Design review of the part built by this model. Coordinates are the model's own, in mm. Face numbers are marked on the shaded views. A direction names the side the tool comes from. Round coordinates to 2 decimals unless told otherwise and drop trailing zeros. Order: outer loops, then holes, each group sorted by start corner. A loop starts at its lowest first (then second) coordinate and runs counter-clockwise, first axis right, second up. Notation, with made-up numbers: (59, -3.75) - (102, -3.75) arc R37 cw to (102, 33.25) - close; hole circle Ø4 at (59, 0.25). An arc over 180 degrees is marked (long way). Write item = value, one per line.
from build123d import *

# Parameters (mm, degrees)
F0_R     = 9.525
F1_DEPTH = 50.8
F2_SIZE  = 0.762
F3_W     = 9.525
F3_H     = 5.747142
F4_DEPTH = 12.7


with BuildPart() as f1:
    # F0 (on Front) → F1 (new body)
    with BuildSketch(Plane.XZ):
        Circle(F0_R)
    extrude(amount=-F1_DEPTH)

    # F2
    f2_edges = [f1.edges().sort_by_distance(p)[0] for p in [
        (-9.525, 0, 0),
        (-9.525, 50.8, 0),
    ]]
    chamfer(f2_edges, length=F2_SIZE)

    # F3 (on Right) → F4 (cut, symmetric)
    with BuildSketch(Plane.YZ):
        with Locations((12.7, 9.223571)):
            Rectangle(F3_W, F3_H)
        with Locations((38.1, 9.223571)):
            Rectangle(F3_W, F3_H)
    extrude(amount=F4_DEPTH, both=True, mode=Mode.SUBTRACT)


solid = f1.part
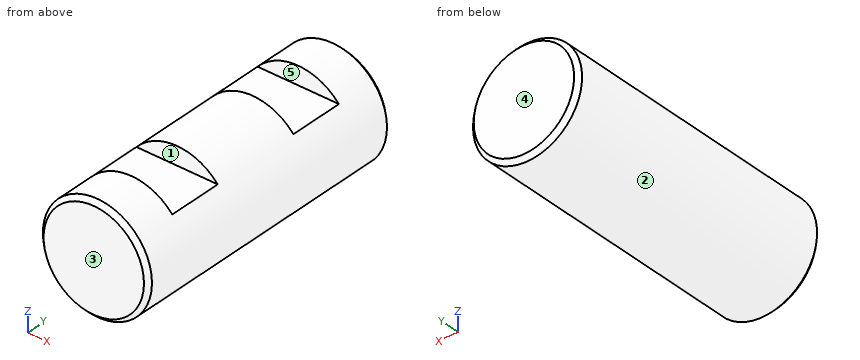
Item 1: Insertion check: P1, Ø3, axis at x = -7, y = 34, coming from the +Z side; P2, Ø6, axis at x = 3, y = 37.5, coming from the +Z side; P3, Ø2, axis at y = 19, z = 4, coming from the +X side. Each pin has a flat end and moves straight along its axis. Give the tip position at first contact, or say it passes through.
Data:
P1 = 7.67
P2 = 6.35
P3 = 9.04
Item 2: Take a section at B-B, the plane y = 6.5. State the section outline as (x, z) points (3 decimals), and give its area (3 significant figures).
Data:
outline = circle Ø19.05 at (0, 0)
area = 285 mm2
Item 3: For line 1 along Y through (x, z) = (-2.75, 6.75); line 2 along X through (y, z) = (9, -7.5); line 3 along Z through (x, y) = (2, 41), list the stretches that pass through material, from the lowest coordinate up. Write a range as [from, to].
Data:
line_1 = [0, 7.94], [17.46, 33.34], [42.86, 50.8]
line_2 = [-5.87, 5.87]
line_3 = [-9.31, 6.35]
Item 4: For the marked faces 1 and 2, list the 3-axis set-ups (+Z, -Z, +X, -X, +Y, -Y) from which the entire face can be reached by the end or side of a thin tool; tool diameter is ignored.
Data:
face_1 = +Z, +X, -X
face_2 = +Y, -Y
Item 5: The part is to be moulded in two halves that separate along Y. For the marked faces 3, 4 and 5, say which applies: +Y half, -Y half, draft (parallel to the pull), parting line (faces both ways), or undercut.
Data:
face_3 = -Y half
face_4 = +Y half
face_5 = undercut
